Geometry check sheet. Reference: the model listing, model coordinates, mm. A direction names the side the tool comes from. Round coordinates to 2 decimals unless told otherwise and drop trailing zeros. Write each loop counter-clockwise with the first axis right and the second up, starting at its lowest first coordinate (ties: lowest second). Pieces come first, ordered by that corner, then holes. Notation, with made-up numbers: M 66.25,-32 L 108.25,-32 A25 cw 108.25,2 Z; hole C 55.5,61.5 d11. An arc over 180 degrees is marked long. One line per item, written item: value. Start each with the question number.
1. Release check for a two-part mould opening along X. For faces 3 (the flat face through (0, 0, -2)), 4 (the cylindrical face through (7.04, 2.86, -4.1)), 5 (the flat face through (10, 0, -5)) record: pulls with the +X half, pulls with the -X half, needs draft (parallel to the pull), parting line crosses it, or undercut.
2. Section check B-B (z = -5). Record the boundary of the cut face in (x, y), and give its area (3 significant figures).
3. Scan lines: probe 1 along Y at (x, z) = (0, -8.5); probe 2 along X at (y, z) = (-2, -6); probe 3 along Z at (x, y) = (1, -2.5). Record each from-to range of solid material in increasing order. Write a range as [from, to].
4. Section check C-C (x = 5.5). Record the boundary of the cut face in (y, z), and give its area (3 significant figures).
5. Depth check by flat-ended pin: P1, Ø1.8, axis at x = -0.5, y = -1, coming from the -Z side; P2, Ø6, axis at x = 8, z = -3.5, coming from the +Y side; P3, Ø1, axis at x = 2.5, z = -5, coming from the -Y side. Enter the tip coordinate at first touch or a pass-through.
6. Section check A-A (y = 0). Record the boundary of the cut face in (x, z).
7. Access from +Z, -Z, +X, -X, +Y, -Y to the whole of each face (thin tool, end or side, straight path). Record for faces 1 (the flat face through (0, 0, 0)), 2 (the cylindrical face through (0, -3, -6)).
8. Section check D-D (z = -8.75). Record the boundary of the cut face in (x, y).
Autodesk Inventor part; units mm, degrees
ref_plane "Work Plane1" through (10, 0, 0) normal (1, 0, 0) x (0, 1, 0)
ref_plane "XZ Plane" through (0, 0, 0) normal (0, 1, 0) x (-1, 0, 0)
ref_plane "XY Plane" through (0, 0, 0) normal (0, 0, 1) x (1, 0, 0)
sketch "Sketch1" plane through (0, 0, 0) normal (0, 0, 1) x (1, 0, 0)
  circle A0 centre (0, 0) radius 5
  dimension "d0" = 10
extrude "Extrusion1" add sketch "Sketch1" against normal blind 10
sketch "Sketch2" plane through (0, 0, -10) normal (0, 0, -1) x (-1, 0, 0)
  circle A0 centre (0, 0) radius 5
hole "Hole1" at (0, 0, -10) direction (0, 0, 1) diameter 6 depth 8
ref_plane "Work Plane1" through (10, 0, 0) normal (1, 0, 0) x (0, 1, 0)
sketch "Sketch3" plane through (10, 0, 0) normal (1, 0, 0) x (0, 1, 0)
  circle A0 centre (0, -5) radius 3
  line L0 (5, 0) -> (5, -10)
  point P0 (0, 0)
  point P1 (5, -5)
  dimension "d11" = 6
extrude "Extrusion2" add sketch "Sketch3" against normal up to surface
properties part number "verbindungoben"
Result sheet:
1. face 3: undercut
1. face 4: needs draft
1. face 5: pulls with the +X half
2. outline: M 4,-3 L 10,-3 L 10,3 L 4,3 A5 ccw long Z; hole C 0,0 d6
2. area: 82.2 mm2
3. probe 1: y = [-5, -3], [3, 5]
3. probe 2: x = [-4.58, -2.24], [2.24, 10]
3. probe 3: z = [-2, 0]
4. outline: C 0,-5 d6
4. area: 28.3 mm2
5. P1: stops at z = -2
5. P2: stops at y = 3
5. P3: stops at y = -4.58
6. outline: M -5,-10 L -3,-10 L -3,-2 L 3,-2 L 3,-10 L 5,-10 L 5,-8 L 10,-8 L 10,-2 L 5,-2 L 5,0 L -5,0 Z
7. face 1: +Z, +X, -X, +Y, -Y
7. face 2: -Z
8. outline: C 0,0 d10; hole C 0,0 d6
